```python
from build123d import *
from build123d import SkipClean  # not in build123d's __all__

# Parameters (mm, degrees)
F0_W           = 450
F0_H           = 18
F1_DEPTH       = 450
F3_D           = 283
F3_DEPTH       = 36
F3_CBORE_D     = 315
F3_CBORE_DEPTH = 9.7
F3_TIP         = 85.0217775924
F4_R           = 9
F5_R           = 5
F7_D           = 6.6
F7_DEPTH       = 6
F7_TIP         = 1.9828400428
F8_ANGLE       = 180
F9_W           = 414
F9_H           = 396
F9_R           = 141.5
F10_DEPTH      = 18
F13_D          = 13.2
F13_DEPTH      = 25
F13_TIP        = 3.9656800856
F14_D          = 6.6
F14_DEPTH      = 6
F14_TIP        = 1.9828400428


# Not quite as in the source:
# - after a boolean that leaves OpenCascade's solid faulty, fix() repairs it


with BuildPart() as f1:
    # F0 (on Front) → F1 (new body)
    with BuildSketch(Plane.XZ):
        with Locations((-0.2429935762, -1.4711191316)):
            Rectangle(F0_W, F0_H)
    extrude(amount=F1_DEPTH)

    # F3
    with Locations(Plane.XY.offset(7.5288808684)):
        with Locations((-0.2429935762, -225)):
            CounterBoreHole(F3_D / 2, F3_CBORE_D / 2, F3_CBORE_DEPTH, depth=F3_DEPTH)
            with Locations((0, 0, -(F3_DEPTH + F3_TIP / 2))):  # 118° drill point
                Cone(0, F3_D / 2, F3_TIP, mode=Mode.SUBTRACT)

    # F4
    f4_edges = [f1.edges().sort_by_distance(p)[0] for p in [
        (-225.242994, -450, -1.471119),
        (-225.242994, 0, -1.471119),
        (224.757006, 0, -1.471119),
        (224.757006, -450, -1.471119),
    ]]
    fillet(f4_edges, radius=F4_R)

    # F5
    f5_edges = [f1.edges().sort_by_distance(p)[0] for p in [
        (-0.242994, 0, 7.528881),
        (224.757006, -225, 7.528881),
        (-0.242994, -450, 7.528881),
        (-225.242994, -225, 7.528881),
    ]]
    fillet(f5_edges, radius=F5_R)

    # F7
    with Locations(Plane(origin=(0, 0, -10.4711191316), x_dir=(1, 0, 0), z_dir=(0, 0, -1))):
        with Locations((-216.2429935762, 441), (-108.1214967881, 441), (0, 441), (108.1214967881, 441), (216.2429935762, 441), (108.1214967881, 423), (0, 423), (-108.1214967881, 423), (-198.2429935762, 423), (198.2429935762, 423), (216.2429935762, 333), (216.2429935762, 225), (216.2429935762, 117), (216.2429935762, 9), (108.1214967881, 9), (0, 9), (-108.1214967881, 9), (-216.2429935762, 9), (-216.2429935762, 117), (-216.2429935762, 225), (-216.2429935762, 333), (-216.2429935762, 423), (216.2429935762, 423)):
            Hole(F7_D / 2, depth=F7_DEPTH)
            with Locations((0, 0, -(F7_DEPTH + F7_TIP / 2))):  # 118° drill point
                Cone(0, F7_D / 2, F7_TIP, mode=Mode.SUBTRACT)


with BuildPart() as f1_1:
    # F8: moved
    add(f1.part.rotate(Axis((224.7570064238, -225, -10.4711191316), (0, 1, 0)), F8_ANGLE), clean=False)

    # F9 (on face) → F10 (join)
    with BuildSketch(Plane.XY.offset(-10.4711191316)):
        with Locations((449.7570064238, -216)):
            Rectangle(F9_W, F9_H)
        with Locations((449.7570064238, -225)):
            Circle(F9_R, mode=Mode.SUBTRACT)
    with SkipClean():  # cleaning this boolean's faces spoils the solid; the shape is the same uncleaned
        extrude(amount=F10_DEPTH)

    # F13
    with Locations(Plane(origin=(0, 0, -28.4711191316), x_dir=(1, 0, 0), z_dir=(0, 0, -1))):
        with Locations((628.2570064238, 46.5), (271.2570064238, 46.5), (271.2570064238, 403.5), (628.2570064238, 403.5)):
            Hole(F13_D / 2, depth=F13_DEPTH)
            with Locations((0, 0, -(F13_DEPTH + F13_TIP / 2))):  # 118° drill point
                Cone(0, F13_D / 2, F13_TIP, mode=Mode.SUBTRACT)

    add(f1_1.part.fix(), mode=Mode.REPLACE)

    # F14
    with Locations(Plane.XY.offset(7.5288808684)):
        with Locations((262.7570064238, -225), (636.7570064238, -225)):
            Hole(F14_D / 2, depth=F14_DEPTH)
            with Locations((0, 0, -(F14_DEPTH + F14_TIP / 2))):  # 118° drill point
                Cone(0, F14_D / 2, F14_TIP, mode=Mode.SUBTRACT)


solid = f1_1.part
```
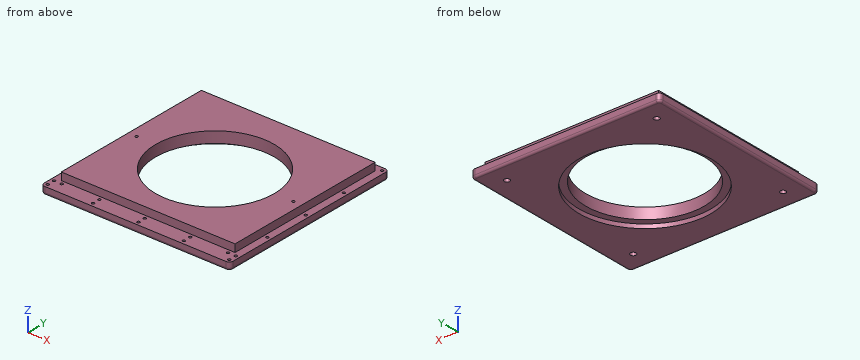
Can you work these out from the model? Positions are in its coordinate system, mm. Give positions to 0.01 mm unless a question says otherwise; leave off trailing zeros. Loops run counter-clockwise (first coordinate to the right, second up) from the corner with the lowest first, then second, coordinate; pieces in that order, holes last. Notation, with made-up numbers: M -9.5,-17.75 L 48.5,-17.75 A22 cw 48.5,17.25 Z; hole C 52,3.25 d7. An arc over 180 degrees is marked long. Use one line per item in the form item = value. Start each with the question number.
(1) Please list where these lines run through material, in increasing order: line 1 (X direction, y = -441, z = -13); line 2 (X direction, y = -333, z = -14.5); line 3 (Y direction, x = 244, z = -0.5).
(2) I'm going to push flat-ended pins straight in: P1, Ø5.5, axis at x = 251.27, y = -423, coming from the +Z side; P2, Ø8, axis at x = 271.26, y = -46.5, coming from the -Z side; P3, Ø1.5, axis at y = -355.5, z = -3, coming from the -X side. Where does each tip first touch, or does it pass through?
(3) I want a section at B-B, the plane x = 416.5. Write out the boundary of the cut face in (y, z), and give its area (3 significant figures).
(4) I want a section at A-A, the plane y = -97. Write out the boundary of the cut face in (x, z).
Worked out:
q1.line_1 = 224.76 to 229.97, 236.57 to 338.09, 344.69 to 446.21, 452.81 to 554.34, 560.94 to 662.46, 669.06 to 674.76
q1.line_2 = 224.76 to 229.97, 236.57 to 358.33, 541.18 to 662.46, 669.06 to 674.76
q1.line_3 = -414 to -18
q2.P1 = -16.8
q2.P2 = -1.91
q2.P3 = 242.76
q3.outline = M -450,-23.47 A5 ccw -445,-28.47 L -378.95,-28.47 L -378.95,-18.77 L -362.54,-18.77 L -362.54,7.53 L -414,7.53 L -414,-10.47 L -450,-10.47 Z; M -87.46,-18.77 L -71.05,-18.77 L -71.05,-28.47 L -5,-28.47 A5 ccw 0,-23.47 L 0,-10.47 L -18,-10.47 L -18,7.53 L -87.46,7.53 Z
q3.area = 5,000 mm²
q4.outline = M 224.76,-23.47 A5 ccw 229.76,-28.47 L 357.98,-28.47 L 357.98,-18.77 L 389.44,-18.77 L 389.44,7.53 L 242.76,7.53 L 242.76,-10.47 L 224.76,-10.47 Z; M 510.07,-18.77 L 541.53,-18.77 L 541.53,-28.47 L 669.76,-28.47 A5 ccw 674.76,-23.47 L 674.76,-10.47 L 656.76,-10.47 L 656.76,7.53 L 510.07,7.53 Z
